```python
from build123d import *

# Parameters (mm, degrees)
SKETCH1_W           = 165
SKETCH1_H           = 80
BOSS_EXTRUDE1_DEPTH = 10
SKETCH2_W           = 20
SKETCH2_H           = 80
BOSS_EXTRUDE2_DEPTH = 50
CUT_EXTRUDE1_REACH  = 106.433
SKETCH3_R           = 5


with BuildPart() as part:
    # Sketch1 → Boss-Extrude1 (new body)
    with BuildSketch(Plane.XY):
        Rectangle(SKETCH1_W, SKETCH1_H)
    extrude(amount=BOSS_EXTRUDE1_DEPTH)

    # Sketch2 → Boss-Extrude2 (add)
    with BuildSketch(Plane.XY.offset(10)):
        with Locations((-72.5, 0)):
            Rectangle(SKETCH2_W, SKETCH2_H)
    extrude(amount=BOSS_EXTRUDE2_DEPTH)

    # Sketch3 → Cut-Extrude1 (cut, up to next)
    with BuildSketch(Plane.XY.offset(10), mode=Mode.PRIVATE) as cut_extrude1_sk1:
        Circle(SKETCH3_R)
    cut_extrude1_tool1 = extrude(cut_extrude1_sk1.sketch, amount=-CUT_EXTRUDE1_REACH, mode=Mode.PRIVATE) & part.part
    add(cut_extrude1_tool1.solids().sort_by_distance((0, 0, 10))[0], mode=Mode.SUBTRACT)


solid = part.part
```
Can you work these out from the model? Positions are in its coordinate system, mm. Give positions to 0.01 mm unless a question says otherwise; leave off trailing zeros. Write each loop counter-clockwise with the first axis right and the second up, starting at its lowest first coordinate (ties: lowest second). Pieces come first, ordered by that corner, then holes. Notation, with made-up numbers: (-34.75, 36) - (16.25, 36) arc R16 cw to (16.25, 50) - close; hole circle Ø2 at (12, -2.5). An arc over 180 degrees is marked (long way). Write item = value, one per line. Start each with the question number.
1. Imagine slicing it at D-D (z = 50.5). Please give me the cut outline in (x, y).
2. Imagine slicing it at A-A (y = 0). Please give me the cut outline in (x, z).
3. Imagine slicing it at B-B (x = 0). Please give me the cut outline in (y, z), and give its area (3 significant figures).
4. For pin 1 (5 mm diameter, centred on x = 65.5, y = -17, fed in from -Z); pin 2 (25 mm diameter, centred on y = -5.5, z = 36, fed in from +X); pin 3 (1 mm diameter, centred on x = 37, y = -18, fed in from +Z), each with a flat end and sliding along its axis, tell me the tip position at first contact or that it passes through.
5. Imagine slicing it at C-C (y = 9.5). Please give me the cut outline in (x, z), and give its area (3 significant figures).
6. Please list where these lines run through material, in increasing order: line 1 (Y direction, x = 0, z = 4.5); line 2 (Z direction, x = 12.5, y = 6); line 3 (X direction, y = 27, z = 16).
7. Thinking about a two-plate mould opening in X: for faces 1 (the face through (-1.08, -4.88, 5.07)), 2 (the face through (-62.5, -1, 35)), 3 (the face through (9, 1, 10)), which applies, released by +X, released by -X, zero draft, split by the parting line, or undercut?
Worked answers:
q1.outline = (-82.5, -40) - (-62.5, -40) - (-62.5, 40) - (-82.5, 40) - close
q2.outline = (-82.5, 0) - (-5, 0) - (-5, 10) - (-62.5, 10) - (-62.5, 60) - (-82.5, 60) - close; (5, 0) - (82.5, 0) - (82.5, 10) - (5, 10) - close
q3.outline = (-40, 0) - (-5, 0) - (-5, 10) - (-40, 10) - close; (5, 0) - (40, 0) - (40, 10) - (5, 10) - close
q3.area = 700 mm2
q4.pin_1 = 0
q4.pin_2 = -62.5
q4.pin_3 = 10
q5.outline = (-82.5, 0) - (82.5, 0) - (82.5, 10) - (-62.5, 10) - (-62.5, 60) - (-82.5, 60) - close
q5.area = 2,650 mm2
q6.line_1 = -40 to -5, 5 to 40
q6.line_2 = 0 to 10
q6.line_3 = -82.5 to -62.5
q7.face_1 = undercut
q7.face_2 = released by +X
q7.face_3 = zero draft
